Read the model definition and answer for the solid it produces. Units are mm, in the model's axes. Face numbers are marked on the shaded views. Coordinates: 2 decimals unless noted, no trailing zeros. Write each loop counter-clockwise with the first axis right and the second up, starting at its lowest first coordinate (ties: lowest second). Pieces come first, ordered by that corner, then holes. Notation, with made-up numbers: M 41,31.25 L 96,31.25 A17 cw 96,37.25 Z; hole C 39.25,49.25 d7. An arc over 180 degrees is marked long. Write item = value, one per line.
from build123d import *

# Parameters (mm, degrees)
SKETCH1_W           = 94
SKETCH1_H           = 130
BOSS_EXTRUDE1_DEPTH = 9.5
SKETCH2_W           = 90.5
SKETCH2_H           = 126.5
CUT_EXTRUDE1_DEPTH  = 2.5
SKETCH3_W           = 70
SKETCH3_H           = 24
CUT_EXTRUDE2_DEPTH  = 8
SKETCH4_W           = 64
SKETCH4_H           = 77
CUT_EXTRUDE3_DEPTH  = 2
SKETCH5_W           = 23
SKETCH5_H           = 3.5
CUT_EXTRUDE4_DEPTH  = 8.5
SKETCH6_W           = 6
SKETCH6_H           = 18
CUT_EXTRUDE5_DEPTH  = 3.5
SKETCH7_W           = 43
SKETCH7_H           = 7.5
CUT_EXTRUDE6_DEPTH  = 3
FILLET1_R           = 2


with BuildPart() as part:
    # Sketch1 → Boss-Extrude1 (new body)
    with BuildSketch(Plane(origin=(0, 7, 0), x_dir=(1, 0, 0), z_dir=(0, 1, 0))):
        with Locations((47, 65)):
            Rectangle(SKETCH1_W, SKETCH1_H)
    extrude(amount=-BOSS_EXTRUDE1_DEPTH)

    # Sketch2 → Cut-Extrude1 (cut)
    with BuildSketch(Plane.XZ.offset(2.5)):
        with Locations((47, -65)):
            Rectangle(SKETCH2_W, SKETCH2_H)
    extrude(amount=-CUT_EXTRUDE1_DEPTH, mode=Mode.SUBTRACT)

    # Sketch3 → Cut-Extrude2 (cut, through all)
    with BuildSketch(Plane.XZ):
        with Locations((47, -100)):
            Rectangle(SKETCH3_W, SKETCH3_H)
    extrude(amount=-CUT_EXTRUDE2_DEPTH, mode=Mode.SUBTRACT)

    # Sketch4 → Cut-Extrude3 (cut)
    with BuildSketch(Plane(origin=(0, 7, 0), x_dir=(-1, 0, 0), z_dir=(0, 1, 0))):
        with Locations((-47, -44.5)):
            Rectangle(SKETCH4_W, SKETCH4_H)
    extrude(amount=-CUT_EXTRUDE3_DEPTH, mode=Mode.SUBTRACT)

    # Sketch5 → Cut-Extrude4 (cut, through all)
    with BuildSketch(Plane(origin=(0, 5, 0), x_dir=(-1, 0, 0), z_dir=(0, 1, 0))):
        with Locations((-42, -9.25)):
            Rectangle(SKETCH5_W, SKETCH5_H)
    extrude(amount=-CUT_EXTRUDE4_DEPTH, mode=Mode.SUBTRACT)

    # Sketch6 → Cut-Extrude5 (cut)
    with BuildSketch(Plane.XZ):
        with Locations((85, -100)):
            Rectangle(SKETCH6_W, SKETCH6_H)
    extrude(amount=-CUT_EXTRUDE5_DEPTH, mode=Mode.SUBTRACT)

    # Sketch7 → Cut-Extrude6 (cut)
    with BuildSketch(Plane.XZ):
        with Locations((33.5, -115.75)):
            Rectangle(SKETCH7_W, SKETCH7_H)
    extrude(amount=-CUT_EXTRUDE6_DEPTH, mode=Mode.SUBTRACT)

    # Fillet1
    fillet1_edges = [part.edges().sort_by_distance(p)[0] for p in [
        (94, 7, -65),
        (47, 7, 0),
        (0, 7, -65),
        (47, 7, -130),
        (94, 2.25, -130),
        (94, 2.25, 0),
        (0, 2.25, 0),
        (0, 2.25, -130),
    ]]
    fillet(fillet1_edges, radius=FILLET1_R)


solid = part.part
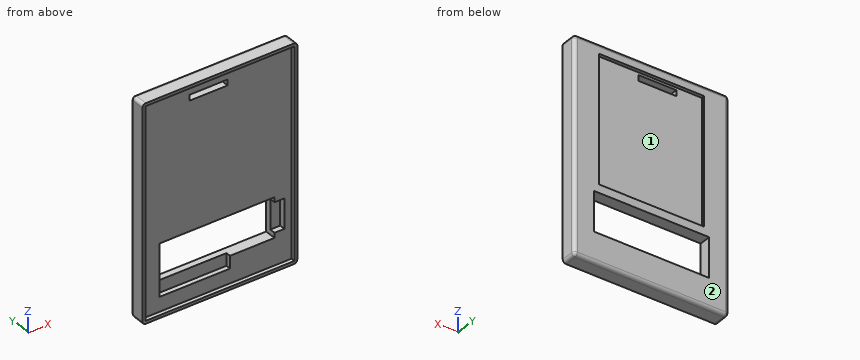
Item 1: Find section B-B (y = 1.5). Determine the outline of the cut face in (x, z).
Worked answers:
outline = M 0,-128 A2 ccw 2,-130 L 92,-130 A2 ccw 94,-128 L 94,-2 A2 ccw 92,0 L 2,0 A2 ccw 0,-2 Z; hole M 12,-119.5 L 55,-119.5 L 55,-112 L 82,-112 L 82,-109 L 88,-109 L 88,-91 L 82,-91 L 82,-88 L 12,-88 Z; hole M 30.5,-11 L 53.5,-11 L 53.5,-7.5 L 30.5,-7.5 Z
Item 2: Find section C-C (z = -107). Determine the outline of the cut face in (x, y), and give its area (3 significant figures).
Worked answers:
outline = M 0,-2.5 L 1.75,-2.5 L 1.75,0 L 12,0 L 12,7 L 2,7 A2 ccw 0,5 Z; M 82,3.5 L 88,3.5 L 88,0 L 92.25,0 L 92.25,-2.5 L 94,-2.5 L 94,5 A2 ccw 92,7 L 82,7 Z
area = 154 mm²
Item 3: Flat-ended cylindrical pins translate along their axes: pin 1 (2 mm diameter, centred on y = 6, z = -31, fed in from -X); pin 2 (1.5 mm diameter, centred on x = 70.5, z = -56, fed in from +Y); pin 3 (5 mm diameter, centred on x = 42, z = -23.5, fed in from -Y). Find the tip coordinate at first contact, or state that the pin passes through.
Worked answers:
pin_1 = 0
pin_2 = 5
pin_3 = 0
Item 4: Find section A-A (x = 28). Determine the outline of the cut face in (y, z).
Worked answers:
outline = M -2.5,-130 L 5,-130 A2 ccw 7,-128 L 7,-112 L 3,-112 L 3,-119.5 L 0,-119.5 L 0,-128.25 L -2.5,-128.25 Z; M -2.5,-1.75 L 0,-1.75 L 0,-88 L 7,-88 L 7,-83 L 5,-83 L 5,-6 L 7,-6 L 7,-2 A2 ccw 5,0 L -2.5,0 Z
Item 5: For a pull along X with two mould halves and no side action, classify the marked faces 1 and 2 as released by +X, released by -X, zero draft, split by the parting line, or undercut.
Worked answers:
face_1 = undercut
face_2 = zero draft
Item 6: Consider line 1 along Z through (x, y) = (45.5, 0.25); line 2 along Z through (x, y) = (53, 4.25); line 3 along Z through (x, y) = (18.5, -0.75). Determine where each line is inside the solid, lowest interval first. Write a range as from..to.
Worked answers:
line_1 = -130..-119.5, -88..-11, -7.5..0
line_2 = -130..-112, -88..-11, -7.5..0
line_3 = -130..-128.25, -1.75..0
Item 7: Find section D-D (x = 48). Determine the outline of the cut face in (y, z), and give its area (3 significant figures).
Worked answers:
outline = M -2.5,-130 L 5,-130 A2 ccw 7,-128 L 7,-112 L 3,-112 L 3,-119.5 L 0,-119.5 L 0,-128.25 L -2.5,-128.25 Z; M -2.5,-1.75 L 0,-1.75 L 0,-7.5 L 5,-7.5 L 5,-6 L 7,-6 L 7,-2 A2 ccw 5,0 L -2.5,0 Z; M 0,-88 L 7,-88 L 7,-83 L 5,-83 L 5,-11 L 0,-11 Z
area = 555 mm²
